from build123d import *

# Parameters (mm, degrees)
SKETCH_3_R               = 7.5
EXTRUDE_2_DEPTH          = 33
SKETCH_4_R               = 5
CUT_EXTRUDE_1_DEPTH      = 15
PATTERN_CIRCULAR_2_COUNT = 4


with BuildPart() as part:
    # 草图2 → 旋转2 (revolve)
    with BuildSketch(Plane.XY, mode=Mode.PRIVATE) as revolve_2_sk:
        with BuildLine():
            Line((-16, 0), (-16, -35))
            Line((-16, -35), (-14, -35))
            Line((-14, -35), (-14, 0))
            Line((-14, 0), (0, 0))
            Line((0, 0), (0, 16))
            ThreePointArc((0, 16), (-11.313708499, 11.313708499), (-16, 0))
        make_face()
    revolve(revolve_2_sk.sketch.rotate(Axis((0, 0, 0), (0, -1, 0)), 270), axis=Axis((0, 0, 0), (0, -1, 0)))

    # 草图3 → 凸台-拉伸2 (add)
    with BuildSketch(Plane.XY):
        with Locations(Location((0, -10, 0), (0, 0, 90.000000001))):
            Circle(SKETCH_3_R)
    extrude_2 = extrude(amount=EXTRUDE_2_DEPTH)

    # 草图4 → 切除-拉伸1 (cut)
    with BuildSketch(Plane.XY.offset(33)):
        with Locations((0, -10)):
            Circle(SKETCH_4_R)
    cut_extrude_1 = extrude(amount=-CUT_EXTRUDE_1_DEPTH, mode=Mode.SUBTRACT)

    # 阵列(圆周)2: 凸台-拉伸2, 切除-拉伸1 ×4 about axis
    pattern_circular_2_axis = Axis((0, 0, 0), (0, 1, 0))
    add([extrude_2.rotate(pattern_circular_2_axis, i * 360 / PATTERN_CIRCULAR_2_COUNT) for i in range(1, PATTERN_CIRCULAR_2_COUNT)])
    add([cut_extrude_1.rotate(pattern_circular_2_axis, i * 360 / PATTERN_CIRCULAR_2_COUNT) for i in range(1, PATTERN_CIRCULAR_2_COUNT)], mode=Mode.SUBTRACT)


solid = part.part
Geometry: final body of the model. Coordinates: model frame, mm. A direction names the side the tool comes from. Round coordinates to 2 decimals unless told otherwise and drop trailing zeros. Order: outer loops, then holes, each group sorted by start corner. A loop starts at its lowest first (then second) coordinate and runs counter-clockwise, first axis right, second up. Notation, with made-up numbers: (80.5, 4.25) - (91.5, 4.25) arc R27 cw to (91.5, 31.25) - close; hole circle Ø7 at (40, 34.25). An arc over 180 degrees is marked (long way). Write each question's results on one line, items separated by ' | '.
Item 1: Section C-C, the plane z = 11. Return the cut outline in (x, y), and give its area (3 significant figures).
Completed:
outline: (-11.62, -35) - (-8.66, -35) - (-8.66, 0) - (8.66, 0) - (8.66, -35) - (11.62, -35) - (11.62, 0) arc R11.62 ccw to (-11.62, 0) - close; circle Ø15 at (0, -10) | area: 596 mm^2
Item 2: Section B-B, the plane z = 21. Return the cut outline in (x, y), and give its area (3 significant figures).
Completed:
outline: circle Ø15 at (0, -10); hole circle Ø10 at (0, -10) | area: 98.2 mm^2
Item 3: First-contact query: pin 1 Ø14 at (x, z) = (-3, -3.5) entering from -Y; pin 2 Ø3 at (x, y) = (-25, -10) entering from +Z; pin 3 Ø1 at (x, y) = (24, -6) entering from -Z. Flat tips, straight axial feed; report the tip coordinate or a pass-through.
Completed:
pin 1: y = -17.5 | pin 2: z = 7.5 | pin 3: z = -6.63
Item 4: Reachability of faces 1 (the cylindrical face through (4.564, -15.952, 8.458)), 2 (the cylindrical face through (0.651, -5.043, -25.605)), 3 (the flat face through (18, -10, 0)), 4 (the cylindrical face through (-23.43, -3.07, 2.87)) from +Z, -Z, +X, -X, +Y, -Y: full face, straight path, thin tool, end or side. Return the list, or none.
Completed:
face 1: none | face 2: -Z | face 3: +X | face 4: -X
Item 5: Section D-D, the plane y = -30. Return the cut outline in (x, z).
Completed:
outline: circle Ø32 at (0, 0); hole circle Ø28 at (0, 0)
Item 6: Mould query, pull axis Y, two halves, no side actions, for faces 5 (the flat face through (0, -10, -18)), 6 (the flat face through (-33, -8, 5)), 7 (the cylindrical face through (-0.651, -5.043, 25.605)), 8 (the cylindrical face through (-2.253, -2.846, 23.435)). Classes: pulls with the +Y half, pulls with the -Y half, needs draft (parallel to the pull), parting line crosses it, or undercut.
Completed:
face 5: undercut | face 6: needs draft | face 7: undercut | face 8: parting line crosses it
Item 7: Material intervals for line 1 along Y through (x, z) = (-26.5, 0); line 2 along Z through (x, y) = (-9.5, -16); line 3 along X through (y, z) = (-13.5, -9), sorted ascending. Write a range as [from, to].
Completed:
line 1: [-17.5, -15], [-5, -2.5] | line 2: [-12.87, -10.28], [-4.5, 4.5], [10.28, 12.87] | line 3: [-13.23, -10.72], [-6.63, 6.63], [10.72, 13.23]
